Could you check a few things on this model? Use its own coordinates, in mm. A direction names the side the tool comes from. Round coordinates to 2 decimals unless told otherwise and drop trailing zeros. Write each loop counter-clockwise with the first axis right and the second up, starting at its lowest first coordinate (ties: lowest second). Pieces come first, ordered by that corner, then holes. Notation, with made-up numbers: (-1, 34.5) - (25, 34.5) arc R28 ccw to (25, 61.5) - close; hole circle Ø4 at (19, 44.25). An arc over 180 degrees is marked (long way). Put each result on its own line as item: value.
from build123d import *

# Parameters (mm, degrees)
SKETCH_1_W          = 54
SKETCH_1_H          = 20
EXTRUDE_1_DEPTH     = 37
SKETCH_2_W          = 67.922695334
SKETCH_2_H          = 39.407561178
SKETCH_2_W_2        = 40
SKETCH_2_H_2        = 20
CUT_EXTRUDE_1_DEPTH = 28
SKETCH_3_W          = 67.922695334
SKETCH_3_H          = 33.385731604
SKETCH_3_W_2        = 40
SKETCH_3_H_2        = 20
CUT_EXTRUDE_2_DEPTH = 6
FILLET_1_R          = 1
FILLET_2_R          = 2
CHAMFER_1_SIZE      = 1
CHAMFER_1_SIZE2     = 2
SKETCH_4_R          = 2
CUT_EXTRUDE_3_DEPTH = 30
RIB_1_REACH         = 48.883
SKETCH_5_WALL_W     = 99.888770984
SKETCH_5_WALL_H     = 1
EXTRUDE_START       = -1
EXTRUDE_4_DEPTH     = 3
SKETCH_9_R          = 6.5
EXTRUDE_5_DEPTH     = 2
CUT_EXTRUDE_START   = -0.5
SKETCH_10_R         = 6.5
SKETCH_10_R_2       = 5
CUT_EXTRUDE_4_DEPTH = 0.5
SKETCH_11_R         = 3
EXTRUDE_6_DEPTH     = 4
SKETCH_14_R         = 1.5
CUT_EXTRUDE_5_DEPTH = 4


with BuildPart() as part:
    # 草图1 → 凸台-拉伸1 (new body)
    with BuildSketch(Plane(origin=(0, 0, 0), x_dir=(1, 0, 0), z_dir=(0, 1, 0))):
        Rectangle(SKETCH_1_W, SKETCH_1_H)
    extrude(amount=EXTRUDE_1_DEPTH)

    # 草图2 → 切除-拉伸1 (cut)
    with BuildSketch(Plane.XZ):
        Rectangle(SKETCH_2_W, SKETCH_2_H)
        Rectangle(SKETCH_2_W_2, SKETCH_2_H_2, mode=Mode.SUBTRACT)
    extrude(amount=-CUT_EXTRUDE_1_DEPTH, mode=Mode.SUBTRACT)

    # 草图3 → 切除-拉伸2 (cut)
    with BuildSketch(Plane(origin=(0, 37, 0), x_dir=(1, 0, 0), z_dir=(0, 1, 0))):
        Rectangle(SKETCH_3_W, SKETCH_3_H)
        Rectangle(SKETCH_3_W_2, SKETCH_3_H_2, mode=Mode.SUBTRACT)
    extrude(amount=-CUT_EXTRUDE_2_DEPTH, mode=Mode.SUBTRACT)

    # 圆角1
    fillet_1_edges = [part.edges().sort_by_distance(p)[0] for p in [
        (20, 14, -10),
        (-20, 14, -10),
        (-20, 14, 10),
        (20, 14, 10),
        (0, 37, -10),
        (0, 37, 10),
        (20, 37, 0),
        (20, 34, 10),
        (-20, 34, 10),
        (-20, 37, 0),
        (-20, 34, -10),
        (20, 34, -10),
    ]]
    fillet(fillet_1_edges, radius=FILLET_1_R)

    # 圆角2
    fillet_2_edges = [part.edges().sort_by_distance(p)[0] for p in [
        (27, 29.5, 10),
        (-27, 29.5, 10),
        (-27, 29.5, -10),
        (27, 29.5, -10),
    ]]
    fillet(fillet_2_edges, radius=FILLET_2_R)

    # 倒角1
    chamfer_1_edges = [part.edges().sort_by_distance(p)[0] for p in [
        (0, 0, -10),
        (0, 0, 10),
        (-20, 0, 0),
        (20, 0, 0),
        (-19.707106781, 0, 9.707106781),
        (19.707106781, 0, 9.707106781),
        (19.707106781, 0, -9.707106781),
        (-19.707106781, 0, -9.707106781),
    ]]
    chamfer_1_side = [part.faces().sort_by_distance(p)[0] for p in [
        (0, 0, 0),
    ]]
    chamfer(chamfer_1_edges, length=CHAMFER_1_SIZE, length2=CHAMFER_1_SIZE2, reference=chamfer_1_side[0])

    # 草图4 → 切除-拉伸3 (cut)
    with BuildSketch(Plane(origin=(0, 37, 0), x_dir=(1, 0, 0), z_dir=(0, 1, 0))):
        with Locations(Location((-24, 5, 0), (0, 0, 270))):
            Circle(SKETCH_4_R)
        with Locations(Location((-24, -5, 0), (0, 0, 270))):
            Circle(SKETCH_4_R)
        with Locations(Location((24, -5, 0), (0, 0, 270))):
            Circle(SKETCH_4_R)
        with Locations(Location((24, 5, 0), (0, 0, 270))):
            Circle(SKETCH_4_R)
    extrude(amount=-CUT_EXTRUDE_3_DEPTH, mode=Mode.SUBTRACT)

    # 草图5 wall → 筋1 (add, up to next)
    with BuildSketch(Plane(origin=(-22, 31.5, 0), x_dir=(-0.970142500145, -0.242535625036, 0), z_dir=(0.242535625036, -0.970142500145, 0)), mode=Mode.PRIVATE) as rib_1_sk1:
        Rectangle(SKETCH_5_WALL_W, SKETCH_5_WALL_H)
    rib_1_tool1 = extrude(rib_1_sk1.sketch, amount=RIB_1_REACH, mode=Mode.PRIVATE) - part.part
    rib_1 = rib_1_tool1.solids().sort_by_distance((-22, 31.5, 0))[0]
    add(rib_1)

    # 镜向1: 筋1 across plane
    add(rib_1.mirror(Plane(origin=(0, 0, 0), x_dir=(0, 0, 1), z_dir=(1, 0, 0))))

    # 草图8 → 凸台-拉伸4 (add)
    with BuildSketch(Plane(origin=(0, 37, 0), x_dir=(1, 0, 0), z_dir=(0, 1, 0)).offset(EXTRUDE_START)):
        with BuildLine():
            Line((-15, 9.5), (6.877501001, 9.5))
            ThreePointArc((6.877501001, 9.5), (20, 0), (6.877501001, -9.5))
            Line((6.877501001, -9.5), (-15, -9.5))
            Line((-15, -9.5), (-15, -3))
            ThreePointArc((-15, -3), (-16, 0), (-15, 3))
            Line((-15, 3), (-15, 9.5))
        make_face()
    extrude(amount=EXTRUDE_4_DEPTH)

    # 草图9 → 凸台-拉伸5 (add)
    with BuildSketch(Plane(origin=(0, 39, 0), x_dir=(1, 0, 0), z_dir=(0, 1, 0))):
        with Locations(Location((10, 0, 0), (0, 0, 270))):
            Circle(SKETCH_9_R)
    extrude(amount=EXTRUDE_5_DEPTH)

    # 草图10 → 切除-拉伸4 (cut)
    with BuildSketch(Plane(origin=(0, 41, 0), x_dir=(1, 0, 0), z_dir=(0, 1, 0)).offset(CUT_EXTRUDE_START)):
        with Locations(Location((10, 0, 0), (0, 0, 270))):
            Circle(SKETCH_10_R)
        with Locations(Location((10, 0, 0), (0, 0, 270))):
            Circle(SKETCH_10_R_2, mode=Mode.SUBTRACT)
    extrude(amount=CUT_EXTRUDE_4_DEPTH, mode=Mode.SUBTRACT)

    # 草图11 → 凸台-拉伸6 (add)
    with BuildSketch(Plane(origin=(0, 41, 0), x_dir=(1, 0, 0), z_dir=(0, 1, 0))):
        with Locations(Location((10, 0, 0), (0, 0, 270))):
            Circle(SKETCH_11_R)
    extrude(amount=EXTRUDE_6_DEPTH)

    # 草图14 → 切除-拉伸5 (cut)
    with BuildSketch(Plane(origin=(0, 45, 0), x_dir=(1, 0, 0), z_dir=(0, 1, 0))):
        with Locations(Location((10, 0, 0), (0, 0, 270))):
            Circle(SKETCH_14_R)
    extrude(amount=-CUT_EXTRUDE_5_DEPTH, mode=Mode.SUBTRACT)


solid = part.part
(1) I'm going to push flat-ended pins straight in: pin 1 (12 mm diameter, centred on y = 13, z = -5, fed in from +X); pin 2 (2.5 mm diameter, centred on x = 17.5, z = 6.5, fed in from +Y); pin 3 (2.5 mm diameter, centred on x = 10, z = 0, fed in from +Y); pin 4 (3.5 mm diameter, centred on x = -24, z = -5, fed in from +Y). Where does each tip first touch, or does it pass through?
Values found:
pin 1: stops at x = 20
pin 2: stops at y = 39
pin 3: stops at y = 41
pin 4: passes through
(2) Imagine slicing it at C-C, the plane y = 29. List the corners of the cut face in (x, z) for me, then the cut area to 3 significant figures.
Values found:
outline: (-27, -8) arc R2 ccw to (-25, -10) - (25, -10) arc R2 ccw to (27, -8) - (27, 8) arc R2 ccw to (25, 10) - (-25, 10) arc R2 ccw to (-27, 8) - close; hole circle Ø4 at (-24, -5); hole circle Ø4 at (-24, 5); hole circle Ø4 at (24, -5); hole circle Ø4 at (24, 5)
area: 1,030 mm^2
(3) If we mould it in two halves opening along X, with no side actions, what happens to faces 4 (the face through (0, 19, 10)), 5 (the face through (-22, 30, -5)), 6 (the face through (-24, 30, 3)), 7 (the face through (-26.4, 29.52, 9.43))? For each: pulls with the +X half, pulls with the -X half, needs draft (parallel to the pull), parting line crosses it, or undercut.
Values found:
face 4: needs draft
face 5: undercut
face 6: undercut
face 7: pulls with the -X half
(4) Imagine slicing it at A-A, the plane x = -4.5. List the corners of the cut face in (y, z) for me, then the cut area to 3 significant figures.
Values found:
outline: (0, -9) - (2, -10) - (36, -10) arc R1 ccw to (36.87, -9.5) - (39, -9.5) - (39, 9.5) - (36.87, 9.5) arc R1 ccw to (36, 10) - (2, 10) - (0, 9) - close
area: 776 mm^2
(5) For faces 1 (the face through (18, 37, -8)), 2 (the face through (10.1, 41, 3.3)), 3 (the face through (18, 37, 8)), which set-ups out of +Z, -Z, +X, -X, +Y, -Y let a thin tool reach every point of the face, with its end or its side?
Values found:
face 1: -Z, +X, +Y
face 2: +Y
face 3: +Z, +X, +Y
(6) Imagine slicing it at B-B, the plane y = 8.5. List the corners of the cut face in (x, z) for me, then the cut area to 3 significant figures.
Values found:
outline: (-20, -9) arc R1 ccw to (-19, -10) - (19, -10) arc R1 ccw to (20, -9) - (20, 9) arc R1 ccw to (19, 10) - (-19, 10) arc R1 ccw to (-20, 9) - close
area: 799 mm^2
(7) Please list where these lines run through material, in increasing order: probe 1 along X at (y, z) = (28.9, -5); probe 2 along X at (y, z) = (43.6, 0); probe 3 along X at (y, z) = (33, 1.75). Write a range as from..to.
Values found:
probe 1: x = -27..-26, -22..22, 26..27
probe 2: x = 7..8.5, 11.5..13
probe 3: x = -20..20
